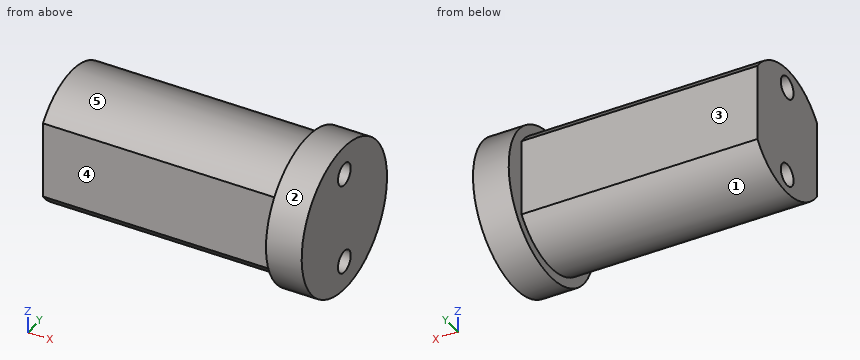
```python
from build123d import *

# Parameters (mm, degrees)
SKETCH_1_R               = 4.15
EXTRUDE_1_DEPTH          = 2
EXTRUDE_2_DEPTH          = 13.2
CUT_EXTRUDE_1_DEPTH      = 15.445933684
CUT_EXTRUDE_1_DEPTH_BACK = 15.445933684
SKETCH_3_R               = 0.619261525


with BuildPart() as part:
    # Эскиз1 → Бобышка-Вытянуть1 (new body)
    with BuildSketch(Plane(origin=(0, 0, 0), x_dir=(0, 0, -1), z_dir=(1, 0, 0))):
        Circle(SKETCH_1_R)
    extrude(amount=EXTRUDE_1_DEPTH)

    # Эскиз2 → Бобышка-Вытянуть2 (add)
    with BuildSketch(Plane.ZY):
        with BuildLine():
            Line((2.133072901, 2.9), (-2.133072901, 2.9))
            ThreePointArc((-2.133072901, 2.9), (-3.6, 0), (-2.133072901, -2.9))
            Line((-2.133072901, -2.9), (2.133072901, -2.9))
            ThreePointArc((2.133072901, -2.9), (3.6, 0), (2.133072901, 2.9))
        make_face()
    extrude(amount=EXTRUDE_2_DEPTH)

    # Эскиз3 → Вырез-Вытянуть1 (cut, two sides: drawn at the far end of the back side and taken through both)
    with BuildSketch(Plane(origin=(0, 0, 0), x_dir=(0, 0, -1), z_dir=(1, 0, 0)).offset(-CUT_EXTRUDE_1_DEPTH_BACK)):
        with Locations((-2.541933221, 0)):
            Circle(SKETCH_3_R)
        with Locations(Location((2.541933221, 0, 0), (0, 0, 180))):
            Circle(SKETCH_3_R)
    extrude(amount=CUT_EXTRUDE_1_DEPTH + CUT_EXTRUDE_1_DEPTH_BACK, mode=Mode.SUBTRACT)


solid = part.part
```
Here's how the part is built. I have some questions about the finished solid (model axes, mm). Face numbers are marked on the shaded views. A direction names the side the tool comes from. Give positions to 0.01 mm unless a question says otherwise; leave off trailing zeros. Loops run counter-clockwise (first coordinate to the right, second up) from the corner with the lowest first, then second, coordinate; pieces in that order, holes last. Notation, with made-up numbers: M 7,85.25 L 12,85.25 A21 cw 12,89.25 Z; hole C 88,66.25 d11. An arc over 180 degrees is marked long. Put each result on its own line as item: value. Start each with the question number.
(1) I want a section at A-A on y = 0. Please give me the cut outline in (x, z).
(2) For the marked faces 1, 2, 3, 4 and 5, which set-ups out of +Z, -Z, +X, -X, +Y, -Y let a thin tool reach every point of the face, with its end or its side?
(3) I want a section at C-C on z = 0. Please give me the cut outline in (x, y).
(4) I want a section at B-B on x = -8.5. Please give me the cut outline in (y, z), then the cut area to 3 significant figures.
(5) I want a section at D-D on y = -1.25. Please give me the cut outline in (x, z), then the cut area to 3 significant figures.
(6) Will these pins go through, and if not, where does the flat tip stop? pin 1 Ø4 at (x, y) = (-2.5, 2.5) entering from -Z; pin 2 Ø3.5 at (x, z) = (-8.5, 0) entering from +Y; pin 3 Ø3 at (x, z) = (-5, 0) entering from -Y.
(7) I need wall thicknesses on line 1 along Z through (x, y) = (-0.5, 0.25); line 2 along X through (y, z) = (0, 3.75); line 3 along Z through (x, y) = (0.5, -0.25). Which ranges of each line are inside material? Lowest first, please. Write a range as [from, to].
Answer block:
1. outline: M -13.2,-3.6 L 0,-3.6 L 0,-4.15 L 2,-4.15 L 2,-3.16 L -13.2,-3.16 Z; M -13.2,-1.92 L 2,-1.92 L 2,1.92 L -13.2,1.92 Z; M -13.2,3.16 L 2,3.16 L 2,4.15 L 0,4.15 L 0,3.6 L -13.2,3.6 Z
2. face 1: -Z, -X
2. face 2: +X, -X
2. face 3: +Z, -Z, -X, +Y
2. face 4: +Z, -Z, -X, -Y
2. face 5: +Z, -X
3. outline: M -13.2,-2.9 L 0,-2.9 L 0,-4.15 L 2,-4.15 L 2,4.15 L 0,4.15 L 0,2.9 L -13.2,2.9 Z
4. outline: M -2.9,-2.13 A3.6 ccw 2.9,-2.13 L 2.9,2.13 A3.6 ccw -2.9,2.13 Z; hole C 0,-2.54 d1.24; hole C 0,2.54 d1.24
4. area: 34.2 mm^2
5. outline: M -13.2,-3.38 L 0,-3.38 L 0,-3.96 L 2,-3.96 L 2,3.96 L 0,3.96 L 0,3.38 L -13.2,3.38 Z
5. area: 105 mm^2
6. pin 1: z = -3.57
6. pin 2: y = 2.9
6. pin 3: y = -2.9
7. line 1: [-3.59, -3.11], [-1.98, 1.98], [3.11, 3.59]
7. line 2: [0, 2]
7. line 3: [-4.14, -3.11], [-1.98, 1.98], [3.11, 4.14]
